```python
from build123d import *

# Parameters (mm, degrees)
F0_W     = 38
F0_H     = 32
F1_DEPTH = 10.1
F0_R     = 1.6
F0_R_2   = 6.35
F2_DEPTH = 1
F3_DEPTH = 10.1


with BuildPart() as f1:
    # F0 (on Front) → F1 (new body)
    with BuildSketch(Plane.XZ):
        Rectangle(F0_W, F0_H)
    extrude(amount=F1_DEPTH)

    # F0 (on Front) → F2 (join)
    with BuildSketch(Plane.XZ):
        with BuildLine():
            ThreePointArc((-35, -20), (-34.12132, -22.12132), (-32, -23))
            Line((-32, -23), (62, -23))
            ThreePointArc((62, -23), (64.12132, -22.12132), (65, -20))
            Line((65, -20), (65, 20))
            ThreePointArc((65, 20), (64.12132, 22.12132), (62, 23))
            Line((62, 23), (-32, 23))
            ThreePointArc((-32, 23), (-34.12132, 22.12132), (-35, 20))
            Line((-35, 20), (-35, -20))
        make_face()
        with Locations((-32, -20)):
            Circle(F0_R, mode=Mode.SUBTRACT)
        with Locations((62, -20)):
            Circle(F0_R, mode=Mode.SUBTRACT)
        Rectangle(F0_W, F0_H, mode=Mode.SUBTRACT)
        with Locations((-32, 20)):
            Circle(F0_R, mode=Mode.SUBTRACT)
        with Locations((48, 0)):
            Circle(F0_R_2, mode=Mode.SUBTRACT)
        with Locations((62, 20)):
            Circle(F0_R, mode=Mode.SUBTRACT)
        Rectangle(F0_W, F0_H)
        with Locations((48, 0)):
            Circle(F0_R_2)
    extrude(amount=-F2_DEPTH)

    # F0 (on Front) → F3 (join, through all)
    with BuildSketch(Plane.XZ):
        with Locations((48, 0)):
            Circle(F0_R_2)
    extrude(amount=F3_DEPTH)


solid = f1.part
```
Part model, mm, in its own coordinate system. A direction names the side the tool comes from. Round coordinates to 2 decimals unless told otherwise and drop trailing zeros. Write each loop counter-clockwise with the first axis right and the second up, starting at its lowest first coordinate (ties: lowest second). Pieces come first, ordered by that corner, then holes. Notation, with made-up numbers: M 20,69 L 72,69 A9 cw 72,73 Z; hole C -27,58 d9. An arc over 180 degrees is marked long. One line per question, with ' | ' between items.
(1) Saw through at B-B on z = 0. Write the cut outline in (x, y).
Answer key:
outline: M -35,0 L -19,0 L -19,-10.1 L 19,-10.1 L 19,0 L 41.65,0 L 41.65,-10.1 L 54.35,-10.1 L 54.35,0 L 65,0 L 65,1 L -35,1 Z
(2) Saw through at A-A on y = -4.25. Write the cut outline in (x, z), then the cut area to 3 significant figures.
Answer key:
outline: M -19,-16 L 19,-16 L 19,16 L -19,16 Z; C 48,0 d12.7 | area: 1,340 mm^2
(3) Saw through at D-D on x = 22.5. Write the cut outline in (y, z).
Answer key:
outline: M 0,-23 L 1,-23 L 1,23 L 0,23 Z
(4) Saw through at C-C on x = 4. Write the cut outline in (y, z), then the cut area to 3 significant figures.
Answer key:
outline: M -10.1,-16 L 0,-16 L 0,-23 L 1,-23 L 1,23 L 0,23 L 0,16 L -10.1,16 Z | area: 369 mm^2
(5) 3-axis set-ups, long thin cutter, end or side, ignore diameter. For faces 4 (the face through (19, -5, 0)), 5 (the face through (0, -5, -16)), 6 (the face through (0, -5, 16)), 7 (the face through (41.656, -4.979, 0.279)): which of +Z, -Z, +X, -X, +Y, -Y reach the whole face in a straight line?
Answer key:
face 4: +Z, -Z, -Y | face 5: -Z, +X, -X, -Y | face 6: +Z, +X, -X, -Y | face 7: -Y
(6) Pin check, flat tips, straight feed: pin 1 (5 mm diameter, centred on x = 4.5, y = -6.5, fed in from +Z); pin 2 (5 mm diameter, centred on y = -5.5, z = 3, fed in from -X); pin 3 (1.5 mm diameter, centred on x = 49, y = -7.5, fed in from +Z). Stop position of each tip, or through.
Answer key:
pin 1: stops at z = 16 | pin 2: stops at x = -19 | pin 3: stops at z = 6.35
(7) Probe line 1 along Z through (x, y) = (-32, 0.2); line 2 along Z through (x, y) = (-2, -0.5); line 3 along X through (y, z) = (-7.5, -7). List the from-to ranges inside material, lowest first.
Answer key:
line 1: z = -23 to -21.6, -18.4 to 18.4, 21.6 to 23 | line 2: z = -16 to 16 | line 3: x = -19 to 19
(8) Two-plate mould, pull along Z, no slides. Class faces 1 (the face through (-19, -5, 0)), 2 (the face through (-33.18, 0.49, -18.92)), 3 (the face through (-34.1, 0.49, 22.14)): released by +Z, released by -Z, zero draft, split by the parting line, or undercut.
Answer key:
face 1: zero draft | face 2: undercut | face 3: released by +Z
